from build123d import *

# Parameters (mm, degrees)
SKETCH_1_R               = 124
SKETCH_1_R_2             = 87
SKETCH_1_R_3             = 10
EXTRUDE_1_DEPTH          = 5
CUT_EXTRUDE_1_DEPTH      = 176.64737402
CUT_EXTRUDE_1_DEPTH_BACK = 176.64737402
SKETCH_2_OUTSIDE_W       = 320.174
SKETCH_2_OUTSIDE_H       = 320.174
SKETCH_2_OUTSIDE_W_2     = 210
SKETCH_2_OUTSIDE_H_2     = 280
CUT_EXTRUDE_2_DEPTH      = 163.791277408
CUT_EXTRUDE_2_DEPTH_BACK = 163.791277408
SKETCH_3_W               = 14
SKETCH_3_H               = 48


with BuildPart() as part:
    # Эскиз1 → Бобышка-Вытянуть1 (new, symmetric)
    with BuildSketch(Plane.XY):
        Circle(SKETCH_1_R)
        Circle(SKETCH_1_R_2, mode=Mode.SUBTRACT)
        with Locations((74.599765415, 74.599765415)):
            Circle(SKETCH_1_R_3, mode=Mode.SUBTRACT)
        with Locations((74.599765415, -74.599765415)):
            Circle(SKETCH_1_R_3, mode=Mode.SUBTRACT)
        with Locations((-74.599765415, -74.599765415)):
            Circle(SKETCH_1_R_3, mode=Mode.SUBTRACT)
        with Locations((-74.599765415, 74.599765415)):
            Circle(SKETCH_1_R_3, mode=Mode.SUBTRACT)
    extrude(amount=EXTRUDE_1_DEPTH, both=True)

    # Эскиз2 outside → Вырез-Вытянуть1 (cut, two sides: drawn at the far end of the back side and taken through both)
    with BuildSketch(Plane.XY.offset(5).offset(-CUT_EXTRUDE_1_DEPTH_BACK)):
        Rectangle(SKETCH_2_OUTSIDE_W, SKETCH_2_OUTSIDE_H)
        Rectangle(SKETCH_2_OUTSIDE_W_2, SKETCH_2_OUTSIDE_H_2, mode=Mode.SUBTRACT)
    extrude(amount=CUT_EXTRUDE_1_DEPTH + CUT_EXTRUDE_1_DEPTH_BACK, mode=Mode.SUBTRACT)

    # Эскиз3 → Вырез-Вытянуть2 (cut, two sides: drawn at the far end of the back side and taken through both)
    with BuildSketch(Plane.XY.offset(5).offset(-CUT_EXTRUDE_2_DEPTH_BACK)):
        with Locations((-66, 124)):
            Rectangle(SKETCH_3_W, SKETCH_3_H)
        with Locations((66, 124)):
            Rectangle(SKETCH_3_W, SKETCH_3_H)
        with Locations((28, 124)):
            Rectangle(SKETCH_3_W, SKETCH_3_H)
        with Locations((-28, 124)):
            Rectangle(SKETCH_3_W, SKETCH_3_H)
    extrude(amount=CUT_EXTRUDE_2_DEPTH + CUT_EXTRUDE_2_DEPTH_BACK, mode=Mode.SUBTRACT)


solid = part.part
Can you work these out from the model? Positions are in its coordinate system, mm. A direction names the side the tool comes from. Give positions to 0.01 mm unless a question says otherwise; leave off trailing zeros. Loops run counter-clockwise (first coordinate to the right, second up) from the corner with the lowest first, then second, coordinate; pieces in that order, holes last. Notation, with made-up numbers: (-12, -17) -> (45, -17) arc R18 cw to (45, -5) -> close; hole circle Ø10 at (9.25, 50.5). An arc over 180 degrees is marked (long way). Write item = value, one per line.
1) Suppose I cut it at C-C on z = 0.5. Write out the boundary of the cut face in (x, y), then the cut area to 3 significant figures.
Check result:
outline = (-105, -65.96) arc R124 ccw to (105, -65.96) -> (105, 65.96) arc R124 ccw to (73, 100.23) -> (73, 100) -> (59, 100) -> (59, 109.06) arc R124 ccw to (35, 118.96) -> (35, 100) -> (21, 100) -> (21, 122.21) arc R124 ccw to (-21, 122.21) -> (-21, 100) -> (-35, 100) -> (-35, 118.96) arc R124 ccw to (-59, 109.06) -> (-59, 100) -> (-73, 100) -> (-73, 100.23) arc R124 ccw to (-105, 65.96) -> close; hole circle Ø174 at (0, 0); hole circle Ø20 at (-74.6, -74.6); hole circle Ø20 at (-74.6, 74.6); hole circle Ø20 at (74.6, -74.6); hole circle Ø20 at (74.6, 74.6)
area = 19,200 mm2
2) Suppose I cut it at B-B on x = 0. Write out the boundary of the cut face in (y, z), then the cut area to 3 significant figures.
Check result:
outline = (-124, -5) -> (-87, -5) -> (-87, 5) -> (-124, 5) -> close; (87, -5) -> (124, -5) -> (124, 5) -> (87, 5) -> close
area = 740 mm2
3) Will these pins go through, and if not, where does the flat tip stop? pin 1 (3 mm diameter, centred on y = 106.5, z = -1, fed in from +X); pin 2 (4 mm diameter, centred on x = 38.5, z = 1.5, fed in from +Y); pin 3 (2 mm diameter, centred on y = -84, z = -3, fed in from +X).
Check result:
pin_1 = 59
pin_2 = 118.51
pin_3 = 92.12
4) Thinking about a two-plate mould opening in X: for faces 1 (the cylindrical face through (90.86, 84.38, 0.07)), 2 (the flat face through (28, 100, 0)), 3 (the flat face through (-105, -1, 0)), which applies, released by +X, released by -X, zero draft, split by the parting line, or undercut?
Check result:
face_1 = released by +X
face_2 = undercut
face_3 = released by -X
5) Suppose I cut it at A-A on y = 0. Write out the boundary of the cut face in (x, z).
Check result:
outline = (-105, -5) -> (-87, -5) -> (-87, 5) -> (-105, 5) -> close; (87, -5) -> (105, -5) -> (105, 5) -> (87, 5) -> close
6) For faces 4 (the cylindrical face through (64.61, -74.16, -0.07)), 5 (the flat face through (35, 109, 0)), which set-ups out of +Z, -Z, +X, -X, +Y, -Y let a thin tool reach every point of the face, with its end or its side?
Check result:
face_4 = +Z, -Z
face_5 = +Z, -Z, +Y
7) Suppose I cut it at D-D on y = 80. Write out the boundary of the cut face in (x, z), then the cut area to 3 significant figures.
Check result:
outline = (-94.74, -5) -> (-83.02, -5) -> (-83.02, 5) -> (-94.74, 5) -> close; (-66.18, -5) -> (-34.19, -5) -> (-34.19, 5) -> (-66.18, 5) -> close; (34.19, -5) -> (66.18, -5) -> (66.18, 5) -> (34.19, 5) -> close; (83.02, -5) -> (94.74, -5) -> (94.74, 5) -> (83.02, 5) -> close
area = 874 mm2
8) I need wall thicknesses on L1, parallel to X at y = 78.5, z = -3.25; L2, parallel to X at y = 80, z = -3.5; L3, parallel to Y at x = 69, z = 4.25. Which ranges of each line are inside material? Lowest first, please. Write a range as from..to.
Check result:
L1 = -95.99..-83.81, -65.39..-37.51, 37.51..65.39, 83.81..95.99
L2 = -94.74..-83.02, -66.18..-34.19, 34.19..66.18, 83.02..94.74
L3 = -103.03..-82.88, -66.31..-52.99, 52.99..66.31, 82.88..100
